Autodesk Inventor part; units mm, degrees
ref_plane "YZ Plane" through (0, 0, 0) normal (1, 0, 0) x (0, 1, 0)
ref_plane "XZ Plane" through (0, 0, 0) normal (0, 1, 0) x (-1, 0, 0)
ref_plane "XY Plane" through (0, 0, 0) normal (0, 0, 1) x (1, 0, 0)
sketch "Sketch1" plane through (0, 0, 0) normal (0, 0, 1) x (1, 0, 0)
  circle A0 centre (8, 0) radius 2.6
  circle A1 centre (-2, 0) radius 2.6
  circle A2 centre (-12, 0) radius 2.6
  line L0 (16, 9.7) -> (16, -9.7)
  line L1 (16, -9.7) -> (-16, -9.7)
  line L2 (-16, -9.7) -> (-16, 9.7)
  line L3 (-16, 9.7) -> (16, 9.7)
  circle A3 centre (-12, 0) radius 2.6
  circle A4 centre (-2, 0) radius 2.6
  circle A5 centre (8, 0) radius 2.6
  line L4 (16, -9.7) -> (-104, -9.7)
  line L5 (-104, -9.7) -> (-104, 9.7)
  line L6 (-104, 9.7) -> (16, 9.7)
  line L7 (16, 9.7) -> (16, -9.7)
  circle A6 centre (-99, -4.7) radius 5
  line L8 (-136.5, 4.5) -> (-136.5, -4.5)
  circle A7 centre (-99, 4.7) radius 5
  point P0 (0, 0)
  point P1 (-126.8, 9.7)
  point P2 (-99, -9.7)
  point P3 (-16, -9.7)
  point P4 (-16, -9.7)
  point P5 (-104, -4.7)
  point P6 (-99, 9.7)
  point P7 (-104, 4.7)
  dimension "d0" = 120
  dimension "d1" = 19.4
  dimension "d18" = 10
extrude "Extrusion1" add sketch "Sketch1" along normal blind 4 contours A0 | A1 | A2 | L0 L1 L2 L3 | L2 L4 A6 A7 L6 | A7 A6 | A6 A7 | A7 A6 L5 | A7 A6
sketch "Sketch11" plane through (0, 0, 0) normal (0, 0, -1) x (-1, 0, 0)
  circle A0 centre (-6.2, 0) radius 5
  line L0 (15, -9.7) -> (15, 9.7)
  circle A1 centre (8, 0) radius 5
  line L1 (-16, -9.7) -> (-16, 9.7)
  point P0 (0, 0)
  dimension "d109" = 10
  dimension "d110" = 10
  dimension "d111" = 9.8
  dimension "d112" = 7
hole "Hole7" at (6.2, 0, 0) at (-8, 0, 0) direction (0, 0, 1) diameter 5.2 depth 5.5
sketch "Sketch12" plane through (0, 0, 0) normal (0, 0, -1) x (-1, 0, 0)
  circle A0 centre (15.636, 0) radius 1.75
  circle A1 centre (35.636, 0) radius 1.75
  circle A2 centre (55.636, 0) radius 1.75
  circle A3 centre (75.636, 0) radius 1.75
  circle A4 centre (95.636, 0) radius 1.75
  point P0 (0, 0)
hole "Hole8" at (-15.636, 0, 0) at (-35.636, 0, 0) at (-55.636, 0, 0) at (-75.636, 0, 0) at (-95.636, 0, 0) direction (0, 0, 1) diameter 2.4 depth 5.5
sketch "Sketch13" plane through (0, 0, 0) normal (0, 0, -1) x (-1, 0, 0)
  circle A0 centre (4, -27.5001) radius 5.25
  circle A1 centre (4, -27.5001) radius 12
  line L0 (-8, -27.5001) -> (-8, -17.7)
  line L1 (99, -9.7) -> (-16, -9.7)
  arc A2 (-8, -17.7) -> (-16, -9.7) centre (-16, -17.7) ccw
  line L2 (4, -39.5001) -> (19, -39.5001)
  arc A3 (19, -39.5001) -> (24, -34.5001) centre (19, -34.5001) ccw
  line L3 (19, -39.5001) -> (19, -34.5001) construction
  line L4 (24, -34.5001) -> (19, -34.5001) construction
  line L5 (24, -34.5001) -> (24, -19.5001)
  arc A4 (33.8001, -9.7) -> (24, -19.5001) centre (33.8001, -19.5001) ccw
  line L6 (-1.6569, -33.1569) -> (9.6569, -21.8432)
  circle A5 centre (4, -27.5001) radius 6
  point P0 (0, 0)
  dimension "d127" = 24
  dimension "d129" = 15
  dimension "d130" = 5
  dimension "d131" = 90
  dimension "d132" = 15
  dimension "d133" = 45
  dimension "d134" = 8
  dimension "d135" = 8
  dimension "d145" = 12
extrude "Extrusion5" add sketch "Sketch13" against normal blind 4
hole "Hole9" at (1.6569, -33.1569, 0) at (-9.6569, -21.8432, 0) direction (0, 0, 1) diameter 3.4 depth 5.5
sketch "Sketch14" plane through (0, 0, 0) normal (0, 0, -1) x (-1, 0, 0)
  line L0 (24, -34.5001) -> (24, -19.5001)
  line L1 (4, -39.5001) -> (19, -39.5001)
  point P0 (0, 0)
  point P1 (20, -35.5001)
  point P2 (20, -15.5001)
  dimension "d146" = 4
  dimension "d147" = 4
  dimension "d148" = 20
hole "Hole10" at (-20, -35.5001, 0) at (-20, -15.5001, 0) direction (0, 0, 1) diameter 2.4 depth 5.5
equation "\"d135\" = d134"
properties part number "back z support"
Geometry: final body of the model. Coordinates: model frame, mm. A direction names the side the tool comes from. Coordinates: 2 decimals unless noted, no trailing zeros. Order: outer loops, then holes, each group sorted by start corner. A loop starts at its lowest first (then second) coordinate and runs counter-clockwise, first axis right, second up. Notation, with made-up numbers: (-20, 27) -> (-8, 27) arc R23 cw to (-8, 50) -> close; hole circle Ø5 at (77.25, 18). An arc over 180 degrees is marked (long way). Write each question's results on one line, items separated by ' | '. Start each with the question number.
1) Cut plane D-D, the plane x = -48.5. Output: boundary loops of the cut face in (y, z), and give its area (3 significant figures).
2) Material intervals for line 1 along X through (y, z) = (-28, 0.45); line 2 along Y through (x, z) = (-61, 1.85); line 3 along X through (y, z) = (1.5, 3), sorted ascending.
3) Mould query, pull axis X, two halves, no side actions, for faces 3 (the flat face through (8, -23, 2)), 4 (the flat face through (-42, 9.7, 2)), 5 (the cylindrical face through (-5.46, -0.56, 2.03)). Classes: released by +X, released by -X, zero draft, split by the parting line, or undercut.
4) Cut plane C-C, the plane x = 6.2. Output: boundary loops of the cut face in (y, z).
5) First-contact query: pin 1 (1.4 mm diameter, centred on x = -35.636, y = 0, fed in from +Z); pin 2 (1 mm diameter, centred on y = -17.5, z = 3.5, fed in from -X); pin 3 (1.2 mm diameter, centred on y = -24, z = 1.5, fed in from +X); pin 4 (2 mm diameter, centred on y = -29.5, z = 1, fed in from -X). Flat tips, straight axial feed; report the tip coordinate or a pass-through.
6) Set-up query: faces 1 (the cylindrical face through (-94.465, -0.26, 2.028)), 2 (the flat face through (-66, -9.7, 2)). Return all of +Z, -Z, +X, -X, +Y, -Y with unobstructed straight access to the full face (end or side cutting, diameter ignored); none if empty.
7) Cut plane A-A, the plane y = 0. State how many separate pieces and enclosed holes the cut face has, and give its area (3 significant figures).
Checks:
1) outline: (-9.7, 0) -> (9.7, 0) -> (9.7, 4) -> (-9.7, 4) -> close | area: 77.6 mm^2
2) line 1: -24 to -9.98, 1.98 to 7.99 | line 2: -9.7 to 9.7 | line 3: -104 to -10.12, -5.88 to 4.08, 8.32 to 16
3) face 3: released by +X | face 4: zero draft | face 5: undercut
4) outline: (-33.82, 0) -> (-2.6, 0) -> (-2.6, 4) -> (-33.82, 4) -> close; (2.6, 0) -> (9.7, 0) -> (9.7, 4) -> (2.6, 4) -> close
5) pin 1: through | pin 2: x = -24.32 | pin 3: x = 8 | pin 4: x = -24
6) face 1: +Z, -Z | face 2: +Z, -Z, -X, -Y
7) separate pieces: 8 | enclosed holes: 0 | area: 390 mm^2
